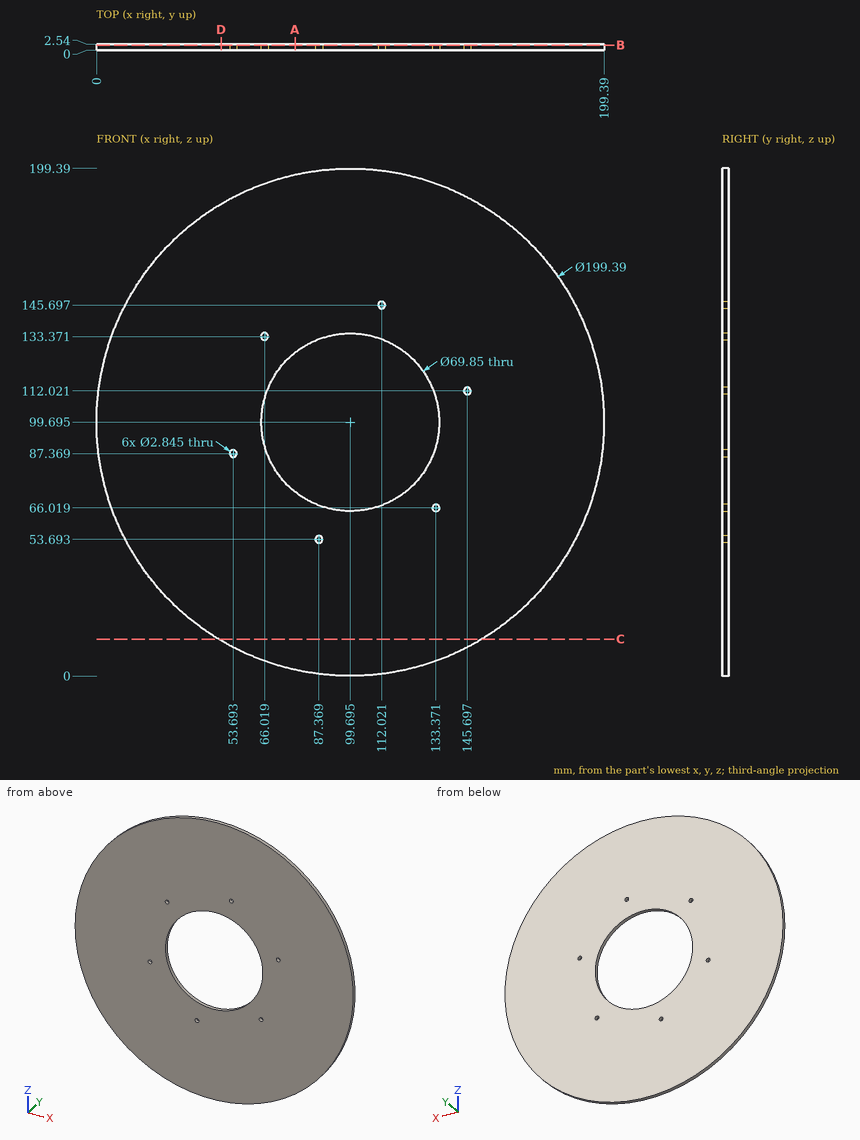
The drawing under review shows one solid part. Ordinate dimensions are in mm from its lowest x, y, z. Coordinates: 2 decimals unless noted, no trailing zeros. Write each loop counter-clockwise with the first axis right and the second up, starting at its lowest first coordinate (ties: lowest second). Pieces come first, ordered by that corner, then holes. Notation, with made-up numbers: (9, 11) -> (46, 11) arc R19 cw to (46, 28) -> close; hole circle Ø6 at (2.25, 89). An arc over 180 degrees is marked (long way). One line per item, written item: value. Start each with the question number.
Q1. Add section A-A, the plane x = 78. Give the boundary of the cut face in (y, z), then the cut area to 3 significant figures.
Q2. To check wall thickness, follow probe 1 along X at (y, z) = (2.15, 100); probe 2 along X at (y, z) = (1.95, 53); probe 3 along Z at (x, y) = (54, 2.35). State the ranges of each line that lie inside material, in increasing order.
Q3. Add section C-C, the plane z = 14.5. Give the boundary of the cut face in (x, y).
Q4. Add section B-B, the plane y = 2.05. Count the separate pieces of the cut face and the enclosed holes in it, then the cut area to 3 significant figures.
Q5. Add section D-D, the plane x = 49. Give the boundary of the cut face in (y, z).
Q6. Clearance check with flat-ended pins moving along their axes: P1, Ø1, axis at x = 37, y = 2, coming from the -Z side; P2, Ø1.5, axis at x = 160.5, y = 1.5, coming from the -Z side; P3, Ø12, axis at x = 118, z = 137, coming from the -Y side; P4, Ø1, axis at y = 1.5, z = 174, coming from the +X side. State where each tip first meets the part, or that it passes through.
Response:
1. outline: (0, 2.39) -> (2.54, 2.39) -> (2.54, 72.33) -> (0, 72.33) -> close; (0, 127.06) -> (2.54, 127.06) -> (2.54, 197) -> (0, 197) -> close
1. area: 355 mm²
2. probe 1: 0 to 64.77, 134.62 to 199.39
2. probe 2: 11.61 to 86.13, 88.61 to 187.78
2. probe 3: 11.09 to 85.98, 88.76 to 188.3
3. outline: (47.92, 0) -> (151.47, 0) -> (151.47, 2.54) -> (47.92, 2.54) -> close
4. separate pieces: 1
4. enclosed holes: 7
4. area: 27,400 mm²
5. outline: (0, 13.85) -> (2.54, 13.85) -> (2.54, 185.54) -> (0, 185.54) -> close
6. P1: z = 21.78
6. P2: z = 20.12
6. P3: y = 0
6. P4: x = 166.72
